from build123d import *

# Parameters (mm, degrees)
SKETCH1_W           = 22.5
SKETCH1_H           = 22.5
BOSS_EXTRUDE1_DEPTH = 2
SKETCH2_W           = 7.5
SKETCH2_H           = 22.5
CUT_EXTRUDE1_DEPTH  = 1
SKETCH4_R           = 1.5
CUT_EXTRUDE2_DEPTH  = 2
SKETCH5_W           = 7.5
SKETCH5_H           = 7.5
CUT_EXTRUDE3_DEPTH  = 2
SKETCH6_R           = 1.5
CUT_EXTRUDE4_DEPTH  = 2
SKETCH7_R           = 1.5
CUT_EXTRUDE5_DEPTH  = 2
FILLET1_R           = 1


with BuildPart() as part:
    # Sketch1 → Boss-Extrude1 (new body)
    with BuildSketch(Plane(origin=(0, 0, 0), x_dir=(1, 0, 0), z_dir=(0, 1, 0))):
        Rectangle(SKETCH1_W, SKETCH1_H)
    extrude(amount=BOSS_EXTRUDE1_DEPTH)

    # Sketch2 → Cut-Extrude1 (cut)
    with BuildSketch(Plane(origin=(0, 2, 0), x_dir=(1, 0, 0), z_dir=(0, 1, 0))):
        Rectangle(SKETCH2_W, SKETCH2_H)
    extrude(amount=-CUT_EXTRUDE1_DEPTH, mode=Mode.SUBTRACT)

    # Sketch4 → Cut-Extrude2 (cut)
    with BuildSketch(Plane(origin=(0, 1, 0), x_dir=(1, 0, 0), z_dir=(0, 1, 0))):
        with Locations(Location((0, 7.5, 0), (0, 0, 270))):
            Circle(SKETCH4_R)
        with Locations(Location((0, -7.5, 0), (0, 0, 270))):
            Circle(SKETCH4_R)
    extrude(amount=-CUT_EXTRUDE2_DEPTH, mode=Mode.SUBTRACT)

    # Sketch5 → Cut-Extrude3 (cut)
    with BuildSketch(Plane(origin=(0, 1, 0), x_dir=(1, 0, 0), z_dir=(0, 1, 0))):
        Rectangle(SKETCH5_W, SKETCH5_H)
    extrude(amount=-CUT_EXTRUDE3_DEPTH, mode=Mode.SUBTRACT)

    # Sketch6 → Cut-Extrude4 (cut)
    with BuildSketch(Plane(origin=(0, 2, 0), x_dir=(1, 0, 0), z_dir=(0, 1, 0))):
        with Locations(Location((-7.5, 7.5, 0), (0, 0, 270))):
            Circle(SKETCH6_R)
        with Locations(Location((-7.5, -7.5, 0), (0, 0, 270))):
            Circle(SKETCH6_R)
        with Locations(Location((-7.5, 0, 0), (0, 0, 270))):
            Circle(SKETCH6_R)
    extrude(amount=-CUT_EXTRUDE4_DEPTH, mode=Mode.SUBTRACT)

    # Sketch7 → Cut-Extrude5 (cut)
    with BuildSketch(Plane(origin=(0, 2, 0), x_dir=(1, 0, 0), z_dir=(0, 1, 0))):
        with Locations(Location((7.5, 0, 0), (0, 0, 270))):
            Circle(SKETCH7_R)
        with Locations(Location((7.5, 7.5, 0), (0, 0, 270))):
            Circle(SKETCH7_R)
        with Locations(Location((7.5, -7.5, 0), (0, 0, 270))):
            Circle(SKETCH7_R)
    extrude(amount=-CUT_EXTRUDE5_DEPTH, mode=Mode.SUBTRACT)

    # Fillet1
    fillet1_edges = [part.edges().sort_by_distance(p)[0] for p in [
        (11.25, 1, 11.25),
        (-11.25, 1, 11.25),
        (-11.25, 1, -11.25),
        (11.25, 1, -11.25),
    ]]
    fillet(fillet1_edges, radius=FILLET1_R)


solid = part.part
For this review, take the finished solid that the model builds, in its own axes (mm). A direction names the side the tool comes from. Give positions to 0.01 mm unless a question says otherwise; leave off trailing zeros. Write each loop counter-clockwise with the first axis right and the second up, starting at its lowest first coordinate (ties: lowest second). Pieces come first, ordered by that corner, then holes. Notation, with made-up numbers: (84, 53) -> (96, 53) arc R28 cw to (96, 80) -> close; hole circle Ø8 at (72, -37.75). An arc over 180 degrees is marked (long way). Use CSV: the item, a comma, the result in double quotes.
Q1. Take a section at A-A, the plane z = -3. Write out the cut boundary in (x, y), then the cut area to 3 significant figures.
Conclusion:
outline,"(-11.25, 0) -> (-3.75, 0) -> (-3.75, 2) -> (-11.25, 2) -> close; (3.75, 0) -> (11.25, 0) -> (11.25, 2) -> (3.75, 2) -> close"
area,"30.0 mm2"
Q2. Tool access review of faces 1 (the face through (-0.1, 1, 5.8)), 2 (the face through (3.75, 1, 0)), 3 (the face through (-0.1, 0.5, 3.75)): name each direction out of +Z, -Z, +X, -X, +Y, -Y from which nothing blocks a thin tool from reaching the whole face with its end or side.
Conclusion:
face 1,"+Z, -Z, +Y"
face 2,"+Y"
face 3,"+Y, -Y"
Q3. For P1, Ø2.5, axis at x = 7.5, z = 7.5, coming from the +Y side; P2, Ø4, axis at x = 7.5, z = -7.5, coming from the +Y side; P3, Ø2, axis at x = 1.5, z = 9.5, coming from the +Y side, all flat-tipped, find the tip position at first contact; note any pin that passes through.
Conclusion:
P1,"through"
P2,"y = 2"
P3,"y = 1"
Q4. Take a section at B-B, the plane x = -2. Write out the cut boundary in (y, z).
Conclusion:
outline,"(0, -11.25) -> (1, -11.25) -> (1, -3.75) -> (0, -3.75) -> close; (0, 3.75) -> (1, 3.75) -> (1, 11.25) -> (0, 11.25) -> close"
Q5. Take a section at D-D, the plane z = 7.5. Write out the cut boundary in (x, y), then the cut area to 3 significant figures.
Conclusion:
outline,"(-11.25, 0) -> (-9, 0) -> (-9, 2) -> (-11.25, 2) -> close; (-6, 0) -> (-1.5, 0) -> (-1.5, 1) -> (-3.75, 1) -> (-3.75, 2) -> (-6, 2) -> close; (1.5, 0) -> (6, 0) -> (6, 2) -> (3.75, 2) -> (3.75, 1) -> (1.5, 1) -> close; (9, 0) -> (11.25, 0) -> (11.25, 2) -> (9, 2) -> close"
area,"22.5 mm2"
Q6. To check wall thickness, follow probe 1 along X at (y, z) = (0.65, 7.5); probe 2 along X at (y, z) = (0.8, 0); probe 3 along X at (y, z) = (1.05, -2.75). State the ranges of each line that lie inside material, in increasing order. Write a range as [from, to].
Conclusion:
probe 1,"[-11.25, -9], [-6, -1.5], [1.5, 6], [9, 11.25]"
probe 2,"[-11.25, -9], [-6, -3.75], [3.75, 6], [9, 11.25]"
probe 3,"[-11.25, -3.75], [3.75, 11.25]"
Q7. Mouldability with a two-part tool opening along X and no side actions: class faces 4 (the face through (10.949, 1.014, -10.965)), 5 (the face through (-0.1, 0.5, -3.75)), 6 (the face through (6.6, 1, -8.7)), 7 (the face through (-11.25, 1, 0)) as pulls with the +X half, pulls with the -X half, needs draft (parallel to the pull), parting line crosses it, or undercut.
Conclusion:
face 4,"pulls with the +X half"
face 5,"undercut"
face 6,"undercut"
face 7,"pulls with the -X half"
Q8. Take a section at C-C, the plane y = 1.35. Write out the cut boundary in (x, z), then the cut area to 3 significant figures.
Conclusion:
outline,"(-11.25, -10.25) arc R1 ccw to (-10.25, -11.25) -> (-3.75, -11.25) -> (-3.75, 11.25) -> (-10.25, 11.25) arc R1 ccw to (-11.25, 10.25) -> close; (3.75, -11.25) -> (10.25, -11.25) arc R1 ccw to (11.25, -10.25) -> (11.25, 10.25) arc R1 ccw to (10.25, 11.25) -> (3.75, 11.25) -> close; hole circle Ø3 at (-7.5, -7.5); hole circle Ø3 at (-7.5, 0); hole circle Ø3 at (-7.5, 7.5); hole circle Ø3 at (7.5, -7.5); hole circle Ø3 at (7.5, 0); hole circle Ø3 at (7.5, 7.5)"
area,"294 mm2"
